Autodesk Fusion 360 part; units mm, degrees
sketch "piston ref" plane through (0, 0, 0) normal (0, 1, 0) x (1, 0, 0)
  circle A0 centre (0, 0) radius 25.35
  circle A1 centre (0, 0) radius 25.55 construction
  dimension "d1" = 50.7
  dimension "d2" = 0.2
  dimension "d3" = 51.1
extrude "Extrude1" add sketch "piston ref" along normal blind 80 makes body 1
sketch "ring mounting" plane through (0, 0, 0) normal (0, 1, 0) x (1, 0, 0)
  circle A0 centre (0, 0) radius 25.55
  line L0 (0, 0) -> (0, 55) construction
  line L1 (0.9964, 28.5326) -> (1.4053, 40.2439)
  line L2 (0, 25.55) -> (0, 40.2684)
  line L3 (0, 40.2684) -> (-4, 40.2684)
  line L4 (-4, 40.2684) -> (-4, 31.5516)
  line L5 (1.4053, 40.2439) -> (5.4029, 40.1043)
  line L6 (5.4029, 40.1043) -> (5.0987, 31.3928)
  line L7 (0.9964, 28.5326) -> (0.8917, 25.5344)
  arc A1 (-7.0169, 27.6743) -> (-4, 31.5516) centre (-8, 31.5516) ccw
  arc A2 (5.0987, 31.3928) -> (7.9784, 27.4125) centre (9.0963, 31.2532) ccw
  line L8 (0, 0) -> (60.8712, -60.8712) construction
  line L9 (0, 0) -> (0, -44) construction
  line L10 (0, -28.55) -> (35.7442, -42.8153)
  line L11 (35.7442, -42.8153) -> (42.8153, -35.7442)
  line L12 (42.8153, -35.7442) -> (28.55, 0)
  line L13 (0, 0) -> (44, 0) construction
  arc A3 (-7.0169, 27.6743) -> (0, -28.55) centre (0, 0) ccw
  arc A4 (28.55, 0) -> (7.9784, 27.4125) centre (0, 0) ccw
  line L14 (18.0666, -18.0666) -> (1.7407, -34.3924) construction
  circle A5 centre (32.2087, -32.2087) radius 3.3
  line L15 (32.2087, -32.2087) -> (47.6032, -16.8142) construction
  point P0 (-4, 28.2684)
  point P1 (4.9841, 28.1116)
  dimension "d8" = 2
  dimension "d9" = 3
  dimension "d10" = 4
  dimension "d11" = 4
  dimension "d14" = 12
  dimension "d15" = 12
  dimension "d16" = 4
  dimension "d31" = 135
  dimension "d32" = 30
  dimension "d33" = 6.6
  dimension "d34" = 10
  dimension "d55" = 20
extrude "Extrude2" add sketch "ring mounting" along normal blind 14 separate body contours A0 L1 L2 L3 L4 L5 L6 L7 A1 A2 L10 L11 L12 A3 A4 makes body 2
sketch "heat insert hole" plane through (3.9976, 0, 0.1396) normal (0.9994, 0, 0.0349) x (0.0349, 0, -0.9994)
  line L0 (31.5516, 0) -> (40.2684, 0)
  line L1 (40.2684, 0) -> (40.2684, 14)
  line L2 (40.2684, 14) -> (31.5516, 14)
  line L3 (31.5516, 14) -> (31.5516, 0)
  circle A0 centre (35.2684, 7) radius 2.3
  line L4 (40.2684, 7) -> (31.5516, 7) construction
  line L5 (35.2684, 14) -> (35.2684, 0) construction
  dimension "d19" = 4.6
  dimension "d30" = 5
extrude "Extrude3" cut sketch "heat insert hole" along direction (-0.996195, 0, -0.087156) blind 4 contours A0 bodies 2
chamfer "Chamfer1" distance 0.4 angle 45 1 edges at (5.1536, 7.8317, -32.9643) on bodies 2
sketch "M3 hole" plane through (-4, 0, 0) normal (-1, 0, 0) x (0, 0, 1)
  line L0 (-40.2684, 0) -> (-31.5516, 0)
  line L1 (-31.5516, 0) -> (-31.5516, 14)
  line L2 (-31.5516, 14) -> (-40.2684, 14)
  line L3 (-40.2684, 14) -> (-40.2684, 0)
  ellipse E0 centre (-35.1073, 7) end of major axis (-35.1073, 9.3) minor radius 2.2986
  circle A0 centre (-35.1073, 7) radius 1.65
  dimension "d24" = 3.3
extrude "Extrude4" cut sketch "M3 hole" against normal blind 4 contours A0 bodies 2
fillet "Fillet1" radius 4 2 edges at (0, 7, -25.55) (0.8917, 7, -25.5344) on bodies 2
chamfer "Chamfer2" distance 0.4 angle 45 4 edges at (5.4029, 7, -40.1043) (1.4053, 7, -40.2439) (0, 7, -40.2684) (-4, 7, -40.2684) on bodies 2
fillet "Fillet2" radius 5 2 edges at (35.7442, 7, 42.8153) (42.8153, 7, 35.7442) on bodies 2
fillet "Fillet3" radius 300 2 edges at (28.55, 7, 0) (0, 7, 28.55) on bodies 2
chamfer "Chamfer6" distance 0.6 angle 45 2 faces at (28.301, 14, 19.6974) (28.301, 0, 19.6974) on bodies 2
chamfer "Chamfer5" [suppressed]
hidden bodies 1
equation "ringDistance = 20 mm"
Verification items for the finished model (mm, model axes). A direction names the side the tool comes from. Coordinates: 2 decimals unless noted, no trailing zeros. One line per item, written item: value.
Item 1: Gauge pin test, flat ends, axial feed: pin 1 Ø3 at (y, z) = (11, -24.5) entering from +X; pin 2 Ø4 at (x, y) = (9.5, 3.5) entering from -Z; pin 3 Ø6.5 at (y, z) = (7, -36) entering from -X. Record the tip position at first contact, or that the pin passes through.
Check sheet entries:
pin 1: stops at x = 16.91
pin 2: stops at z = -27.59
pin 3: stops at x = -4
Item 2: Access from +Z, -Z, +X, -X, +Y, -Y to the whole of each face (thin tool, end or side, straight path). Record for faces 1 (the cylindrical face through (5.877, 6.91, -28.879)), 2 (the flat face through (0, 7, -33)), 3 (the flat face through (-4, 5, -37)), 4 (the cylindrical face through (-1.01, 7.09, -26.62)).
Check sheet entries:
face 1: +X, +Y, -Y
face 2: -Z, +Y, -Y
face 3: -Z, -X, +Y, -Y
face 4: +Y, -Y
Item 3: Scan lines: line 1 along Z through (x, y) = (3, 6.5); line 2 along Z through (x, y) = (2.5, 8.25); line 3 along X through (y, z) = (7, 17). Record each from-to range of solid material in increasing order.
Check sheet entries:
line 1: z = -40.19 to -37.55, -33.05 to -25.67, 25.37 to 30.65
line 2: z = -40.21 to -37.28, -33.41 to -26.01, 25.43 to 30.49
line 3: x = -22.94 to -19.07, 19.07 to 35.44
Item 4: Section check A-A, the plane y = 7. State how many separate pieces and enclosed holes the cut face has, plus the area to 3 significant figures.
Check sheet entries:
separate pieces: 2
enclosed holes: 1
area: 1,210 mm^2
